Geometry check sheet. Reference: the model listing, model coordinates, mm. Face numbers are marked on the shaded views. A direction names the side the tool comes from. Round coordinates to 2 decimals unless told otherwise and drop trailing zeros. Order: outer loops, then holes, each group sorted by start corner. A loop starts at its lowest first (then second) coordinate and runs counter-clockwise, first axis right, second up. Notation, with made-up numbers: (36.25, -25.5) - (84.25, -25.5) arc R28 ccw to (84.25, 4.5) - close; hole circle Ø1 at (49.25, -17.75). An arc over 180 degrees is marked (long way). Answer as CSV lines item,"result". Start each with the question number.
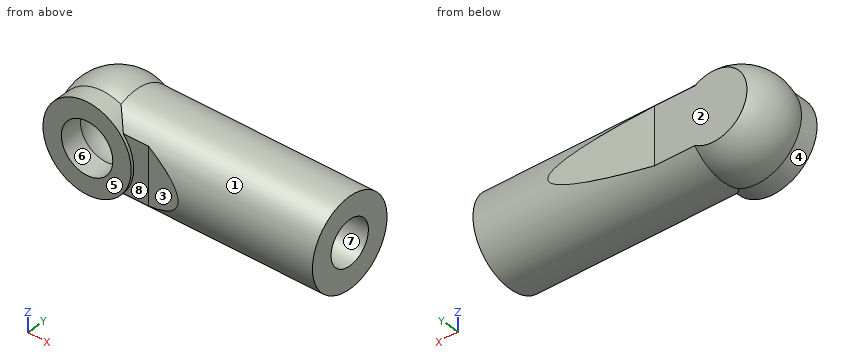
```python
from build123d import *

# Parameters (mm, degrees)
ESQUISSE2_R             = 3
BOSS_EXTRU_1_DEPTH      = 15.75
ESQUISSE3_R             = 1.5
ENL_V_MAT_EXTRU_1_DEPTH = 12
ENL_V_MAT_EXTRU_2_DEPTH = 6
ESQUISSE5_R             = 3
BOSS_EXTRU_2_DEPTH      = 2.5


with BuildPart() as part:
    # Esquisse1 → Révolution1 (revolve)
    with BuildSketch(Plane.XY):
        with BuildLine():
            Line((0, 3.25), (0, -3.25))
            ThreePointArc((0, -3.25), (-3.25, 0), (0, 3.25))
        make_face()
    revolve(axis=Axis((0, 3.25, 0), (0, -1, 0)))

    # Esquisse2 → Boss.-Extru.1 (add)
    with BuildSketch(Plane(origin=(0, 0, 0), x_dir=(0, 0, -1), z_dir=(1, 0, 0))):
        with Locations(Location((0, 0, 0), (0, 0, 180))):
            Circle(ESQUISSE2_R)
    extrude(amount=BOSS_EXTRU_1_DEPTH)

    # Esquisse3 → Enlèv. mat.-Extru.1 (cut)
    with BuildSketch(Plane(origin=(15.75, 0, 0), x_dir=(0, 0, -1), z_dir=(1, 0, 0))):
        Circle(ESQUISSE3_R)
    extrude(amount=-ENL_V_MAT_EXTRU_1_DEPTH, mode=Mode.SUBTRACT)

    # Esquisse4 → Enlèv. mat.-Extru.2 (cut, symmetric)
    with BuildSketch(Plane.XY):
        Polygon((-2.296192501, 2.3), (4, 2.3), (13.038646232, 3.25), (-2.296192501, 3.25), align=None)
        Polygon((-2.296192501, -2.3), (4, -2.3), (7.545448267, -3.25), (-2.296192501, -3.25), align=None)
    extrude(amount=ENL_V_MAT_EXTRU_2_DEPTH, both=True, mode=Mode.SUBTRACT)

    # Esquisse5 → Boss.-Extru.2 (add)
    with BuildSketch(Plane(origin=(0, 0, 0), x_dir=(1, 0, 0), z_dir=(0, 1, 0))):
        with Locations(Location((0, 0, 0), (0, 0, 270))):
            Circle(ESQUISSE5_R)
    extrude(amount=-BOSS_EXTRU_2_DEPTH)

    # Esquisse6 → Enlèvement de matière-Révolution1 (revolve, cut)
    with BuildSketch(Plane.XY):
        with BuildLine():
            Line((1.75, -0.968245837), (1.75, -2.5))
            Line((1.75, -2.5), (0, -2.5))
            Line((0, -2.5), (0, 2))
            ThreePointArc((0, 2), (1.722859784, 1.015753003), (1.75, -0.968245837))
        make_face()
    revolve(axis=Axis((0, -2.5, 0), (0, 1, 0)), mode=Mode.SUBTRACT)


solid = part.part
```
1. Section check B-B on z = 0. Record the boundary of the cut face in (x, y).
2. Go/stop test with flat-tipped pins: pin 1 Ø1.5 at (y, z) = (-1, -1) entering from -X; pin 2 Ø1.5 at (x, z) = (12.5, -1) entering from +Y; pin 3 Ø1.5 at (x, y) = (9.5, 1.5) entering from -Z. Record where each tip stops, or that it passes through.
3. Section check A-A on y = 0. Record the boundary of the cut face in (x, z).
4. Section check C-C on x = 0. Record the boundary of the cut face in (y, z).
5. Section check D-D on x = 11.5. Record the boundary of the cut face in (y, z), plus the area to 3 significant figures.
6. Thickness scan on probe 1 along Z at (x, y) = (0, -1.65); probe 2 along X at (y, z) = (-1.7, 0); probe 3 along Y at (x, z) = (14, 0). Record the ranges inside material, lowest first.
7. Access from +Z, -Z, +X, -X, +Y, -Y to the whole of each face (thin tool, end or side, straight path). Record for the marked faces 1, 2, 3, 4 and 5.
8. Draft check along Y on the marked faces 6, 7 and 8. Enter one of: released by +Y, released by -Y, zero draft, split by the parting line, or undercut.
Numbers:
1,outline,"(-3, -2.5) - (-1.75, -2.5) - (-1.75, -0.97) arc R2 cw (long way) to (1.75, -0.97) - (1.75, -2.5) - (3, -2.5) - (3, -2.3) - (4, -2.3) - (6.61, -3) - (15.75, -3) - (15.75, -1.5) - (3.75, -1.5) - (3.75, 1.5) - (15.75, 1.5) - (15.75, 3) - (10.66, 3) - (4, 2.3) - (-2.3, 2.3) arc R3.25 ccw to (-3, -1.25) - close"
2,pin 1,"stops at x = -3.18"
2,pin 2,"stops at y = 2.99"
2,pin 3,"stops at z = -2.9"
3,outline,"(1.25, -3) - (15.75, -3) - (15.75, -1.5) - (3.75, -1.5) - (3.75, 1.5) - (15.75, 1.5) - (15.75, 3) - (1.25, 3) arc R3.25 ccw (long way) to start; hole circle Ø4 at (0, 0)"
4,outline,"(-2.5, -3) - (-1.25, -3) arc R3.25 ccw to (2.3, -2.3) - (2.3, 2.3) arc R3.25 ccw to (-1.25, 3) - (-2.5, 3) - (-2.5, 1.75) - (-0.97, 1.75) arc R2 cw (long way) to (-0.97, -1.75) - (-2.5, -1.75) - close"
5,outline,"circle Ø6 at (0, 0); hole circle Ø3 at (0, 0)"
5,area,"21.2 mm2"
6,probe 1,"z = -3 to -1.75, 1.75 to 3"
6,probe 2,"x = -3 to -1.75, 1.75 to 15.75"
6,probe 3,"y = -3 to -1.5, 1.5 to 3"
7,face 1,"+X"
7,face 2,"+Z, -Z, -X, +Y"
7,face 3,"+Z, -Z, -Y"
7,face 4,"-Y"
7,face 5,"+Z, -Z, -X, -Y"
8,face 6,"zero draft"
8,face 7,"undercut"
8,face 8,"released by -Y"
